Check sheet for the modelled part. Datum: model origin and axes. Units: mm. Round coordinates to 2 decimals unless told otherwise and drop trailing zeros. Write each loop counter-clockwise with the first axis right and the second up, starting at its lowest first coordinate (ties: lowest second). Pieces come first, ordered by that corner, then holes.
Item 1: Material ranges on line 1 (Y direction, x = 44, z = -1.15); line 2 (Y direction, x = 23.75, z = -2.05); line 3 (Y direction, x = 3, z = -2.5), recorded low to high.
Item 2: Go/stop test with flat-tipped pins: pin 1 Ø1.5 at (y, z) = (34, -1) entering from +X; pin 2 Ø1.5 at (y, z) = (30.5, -1) entering from -X (3 decimals); pin 3 Ø0.9 at (y, z) = (20.5, -2) entering from -X. Record where each tip stops, or that it passes through.
Item 3: Cross-section at A-A on y = 3.5. Enter the section's corners in (x, z), plus the area to 3 significant figures.
Item 4: Cross-section at D-D on y = 22.5. Enter the section's corners in (x, z), plus the area to 4 significant figures.
Item 5: Cross-section at C-C on x = 4. Enter the section's corners in (y, z).
Item 6: Cross-section at B-B on x = 23.75. Enter the section's corners in (y, z).
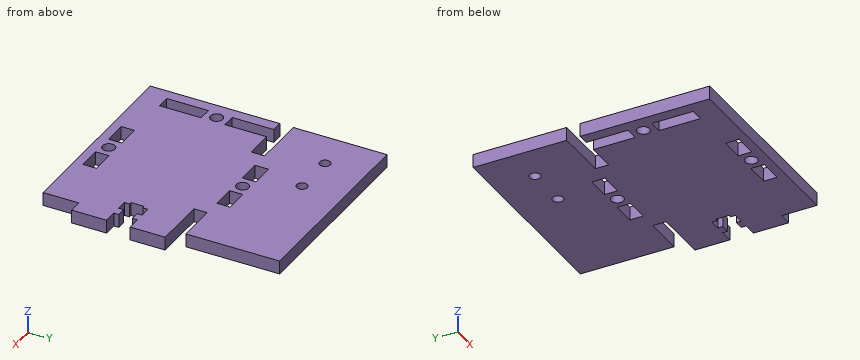
Autodesk Inventor part; units mm, degrees
ref_plane "YZ Plane" through (0, 0, 0) normal (1, 0, 0) x (0, 1, 0)
ref_plane "XZ Plane" through (0, 0, 0) normal (0, 1, 0) x (-1, 0, 0)
ref_plane "XY Plane" through (0, 0, 0) normal (0, 0, 1) x (1, 0, 0)
sketch "Sketch1" plane through (0, 0, 0) normal (0, 0, 1) x (1, 0, 0)
  line L0 (0, 0) -> (47.5, 0)
  line L1 (47.5, 0) -> (47.5, 37)
  line L2 (47.5, 37) -> (0, 37)
  line L3 (0, 37) -> (0, 0)
  dimension "d60" = 47.5
  dimension "d61" = 37
extrude "Extrusion1" add sketch "Sketch1" against normal blind 3
sketch "Sketch6" plane through (0, 0, 0) normal (0, 0, 1) x (1, 0, 0)
  line L0 (47.5, 0) -> (47.5, 37)
  line L1 (47.5, 37) -> (0, 37)
  line L2 (0, 37) -> (47.5, 37)
  line L3 (47.5, 37) -> (44.5, 37)
  line L4 (44.5, 37) -> (44.5, 29)
  line L5 (44.5, 29) -> (47.5, 29)
  line L6 (47.5, 29) -> (47.5, 37)
  line L7 (44.5, 0) -> (44.5, 8)
  line L8 (44.5, 8) -> (47.5, 8)
  line L9 (47.5, 8) -> (47.5, 0)
  line L10 (47.5, 0) -> (44.5, 0)
  line L11 (-10.772, 18.5) -> (61.9279, 18.5) construction
  line L12 (23.75, 42.476) -> (23.75, -8.8223) construction
  line L13 (47.5, 20) -> (39.5, 20)
  line L14 (39.5, 20) -> (39.5, 17)
  line L15 (39.5, 17) -> (47.5, 17)
  line L16 (47.5, 17) -> (47.5, 20)
  line L17 (47.5, 37) -> (47.5, 0)
  line L18 (44.5, 21.15) -> (47.5, 21.15)
  line L19 (47.5, 21.15) -> (47.5, 15.85)
  line L20 (47.5, 15.85) -> (44.5, 15.85)
  line L21 (44.5, 15.85) -> (44.5, 21.15)
  line L22 (40.1, 21.15) -> (42.5, 21.15)
  line L23 (42.5, 21.15) -> (42.5, 15.85)
  line L24 (42.5, 15.85) -> (40.1, 15.85)
  line L25 (40.1, 15.85) -> (40.1, 21.15)
  line L26 (15.8333, 35) -> (21.1, 35)
  line L27 (31.6667, 35) -> (31.6667, 32)
  line L28 (31.6667, 32) -> (26.4, 32)
  line L29 (15.8333, 32) -> (15.8333, 35)
  line L30 (26.4, 35) -> (26.4, 32)
  line L31 (21.1, 32) -> (21.1, 35)
  line L32 (26.4, 35) -> (31.6667, 35)
  line L33 (21.1, 32) -> (15.8333, 32)
  circle A0 centre (23.75, 33.5) radius 1.4
  line L34 (0, 0) -> (47.5, 0)
  line L35 (0, 0) -> (0, 37)
  line L36 (0, 32) -> (11.875, 32)
  line L37 (11.875, 32) -> (11.875, 29)
  line L38 (11.875, 29) -> (0, 29)
  line L39 (0, 29) -> (0, 32)
  line L40 (44.5, 32) -> (35.625, 32)
  line L41 (35.625, 32) -> (35.625, 29)
  line L42 (35.625, 29) -> (44.5, 29)
  line L43 (44.5, 29) -> (44.5, 32)
  line L44 (15.8333, 2) -> (21.1, 2)
  line L45 (31.6667, 2) -> (31.6667, 5)
  line L46 (31.6667, 5) -> (26.4, 5)
  line L47 (15.8333, 5) -> (15.8333, 2)
  line L48 (26.4, 2) -> (26.4, 5)
  line L49 (21.1, 5) -> (21.1, 2)
  line L50 (26.4, 2) -> (31.6667, 2)
  line L51 (21.1, 5) -> (15.8333, 5)
  circle A1 centre (23.75, 3.5) radius 1.4
  line L52 (5.5, 19.65) -> (2.5, 19.65)
  line L53 (2.5, 19.65) -> (2.5, 29)
  line L54 (2.5, 29) -> (5.5, 29)
  line L55 (5.5, 29) -> (5.5, 19.65)
  line L56 (2.5, 14.35) -> (5.5, 14.35)
  line L57 (5.5, 14.35) -> (5.5, 5)
  line L58 (5.5, 5) -> (2.5, 5)
  line L59 (2.5, 5) -> (2.5, 14.35)
  circle A2 centre (4, 17) radius 1.4
  dimension "d65" = 3
  dimension "d75" = 8
  dimension "d76" = 3
  dimension "d78" = 5.3
  dimension "d80" = 5
  dimension "d81" = 2.4
  dimension "d83" = 3
  dimension "d84" = 15.8333
  dimension "d85" = 2
  dimension "d86" = 5.3
  dimension "d87" = 2.8
  dimension "d88" = 3
  dimension "d89" = 23.75
  dimension "d90" = 47.5
  dimension "d91" = 2.8
  dimension "d92" = 5.3
  dimension "d93" = 2.65
  dimension "d94" = 1.5
extrude "Extrusion6" cut sketch "Sketch6" against normal blind 3 contours L10 L7 L8 L0 | L20 L21 L15 L0 | L15 L21 L13 L0 | L35 L36 L37 L38 | L13 L21 L18 L0 | L15 L23 L13 L21 | L38 L55 L52 L53 | L23 L24 L25 L15 | L15 L25 L13 L23 | L5 L4 L1 L0 | L13 L25 L22 L23 | L15 L14 L13 L25 | L42 L41 L40 L4 | L26 L31 L33 L29 | L27 L28 L30 L32 | A0 | L47 L51 L49 L44 | L50 L48 L46 L45 | A1 | L56 L57 L58 L59 | A2
sketch "Sketch9" plane through (0, 37, 0) normal (0, 1, 0) x (1, 0, 0)
  line L0 (44.5, 0) -> (44.5, 3)
  line L1 (0, 3) -> (44.5, 3)
  line L2 (0, 0) -> (0, 3)
  line L3 (44.5, 0) -> (0, 0)
  point P0 (0, 0)
extrude "Extrusion8" add sketch "Sketch9" along normal blind 16
sketch "Sketch10" plane through (0, 0, 0) normal (0, 0, 1) x (1, 0, 0)
  circle A0 centre (8.6339, 43.7833) radius 1.1938
  circle A1 centre (18.1589, 43.7833) radius 1.1938
  line L0 (0, 53) -> (44.5, 53)
  point P0 (0, 0)
  dimension "d99" = 2.3876
  dimension "d100" = 2.3876
  dimension "d101" = 9.2167
  dimension "d102" = 9.2167
extrude "Extrusion9" cut sketch "Sketch10" against normal up to next
equation "\"d89\" = 0.5 * d90"
equation "\"d93\" = 0.5 * d92"
equation "\"d102\" = d101"
equation "\"d15\" = 0.333333 * d14"
properties part number "X-Anchor_Side"
Response values:
1. line 1: y = 0 to 17, 20 to 29, 32 to 53
1. line 2: y = 0 to 2.1, 4.9 to 32.1, 34.9 to 53
1. line 3: y = 0 to 5, 14.35 to 16.02, 17.98 to 19.65, 32 to 53
2. pin 1: stops at x = 44.5
2. pin 2: stops at x = 11.875
2. pin 3: stops at x = 0
3. outline: (0, -3) - (15.83, -3) - (15.83, 0) - (0, 0) - close; (21.1, -3) - (22.35, -3) - (22.35, 0) - (21.1, 0) - close; (25.15, -3) - (26.4, -3) - (26.4, 0) - (25.15, 0) - close; (31.67, -3) - (44.5, -3) - (44.5, 0) - (31.67, 0) - close
3. area: 93.5 mm2
4. outline: (0, -3) - (2.5, -3) - (2.5, 0) - (0, 0) - close; (5.5, -3) - (47.5, -3) - (47.5, 0) - (5.5, 0) - close
4. area: 133.5 mm2
5. outline: (0, -3) - (5, -3) - (5, 0) - (0, 0) - close; (14.35, -3) - (15.6, -3) - (15.6, 0) - (14.35, 0) - close; (18.4, -3) - (19.65, -3) - (19.65, 0) - (18.4, 0) - close; (32, -3) - (53, -3) - (53, 0) - (32, 0) - close
6. outline: (0, -3) - (2.1, -3) - (2.1, 0) - (0, 0) - close; (4.9, -3) - (32.1, -3) - (32.1, 0) - (4.9, 0) - close; (34.9, -3) - (53, -3) - (53, 0) - (34.9, 0) - close
